from build123d import *

# Parameters (mm, degrees)
EXTRUDE_1_DEPTH     = 200
FILLET_1_R          = 80
EXTRUDE_2_DEPTH     = 100
SKETCH_3_R          = 25
CUT_EXTRUDE_1_DEPTH = 160
EXTRUDE_START       = 12
SKETCH_4_R          = 25
EXTRUDE_3_DEPTH     = 12
SKETCH_5_R          = 28
EXTRUDE_4_DEPTH     = 4
SKETCH_6_R          = 20
EXTRUDE_5_DEPTH     = 10
CHAMFER_1_SIZE2     = 5
CHAMFER_1_SIZE      = 10
SKETCH_7_R          = 7
CUT_EXTRUDE_2_DEPTH = 200


with BuildPart() as part:
    # 草图1 → 凸台-拉伸1 (new body)
    with BuildSketch(Plane.XY):
        with BuildLine():
            ThreePointArc((11.613593767, -48.632545068), (50, 0), (11.613593767, 48.632545068))
            Line((11.613593767, 48.632545068), (-48.23619118, 62.924848473))
            Line((-48.23619118, 62.924848473), (-177.193873283, 39.347785035))
            ThreePointArc((-177.193873283, 39.347785035), (-210, 0), (-177.193873283, -39.347785035))
            Line((-177.193873283, -39.347785035), (-48.23619118, -62.924848473))
            Line((-48.23619118, -62.924848473), (11.613593767, -48.632545068))
        make_face()
    extrude(amount=EXTRUDE_1_DEPTH)

    # 圆角1
    fillet_1_edges = [part.edges().sort_by_distance(p)[0] for p in [
        (-48.23619118, -62.924848473, 100),
        (-48.23619118, 62.924848473, 100),
    ]]
    fillet(fillet_1_edges, radius=FILLET_1_R)

    # 草图2 → 凸台-拉伸2 (add)
    with BuildSketch(Plane.XY.offset(200)):
        with BuildLine():
            ThreePointArc((-125, 0), (-132.32233047, 17.67766953), (-150, 25))
            Line((-150, 25), (-150, -25))
            ThreePointArc((-150, -25), (-132.32233047, -17.67766953), (-125, 0))
        make_face()
        with BuildLine():
            Line((-150, -25), (-150, 25))
            ThreePointArc((-150, 25), (-175, 0), (-150, -25))
        make_face()
        with BuildLine():
            Line((-90, 25), (-150, 25))
            ThreePointArc((-150, 25), (-132.32233047, 17.67766953), (-125, 0))
            ThreePointArc((-125, 0), (-132.32233047, -17.67766953), (-150, -25))
            Line((-150, -25), (-90, -25))
            ThreePointArc((-90, -25), (-115, 0), (-90, 25))
        make_face()
        with BuildLine():
            ThreePointArc((-65, 0), (-72.32233047, 17.67766953), (-90, 25))
            Line((-90, 25), (-90, -25))
            ThreePointArc((-90, -25), (-72.32233047, -17.67766953), (-65, 0))
        make_face()
        with BuildLine():
            Line((-90, -25), (-90, 25))
            ThreePointArc((-90, 25), (-115, 0), (-90, -25))
        make_face()
    extrude(amount=EXTRUDE_2_DEPTH)

    # 草图3 → 切除-拉伸1 (cut)
    with BuildSketch(Plane(origin=(0, 0, 0), x_dir=(-1, 0, 0), z_dir=(0, 0, -1))):
        Circle(SKETCH_3_R)
    extrude(amount=-CUT_EXTRUDE_1_DEPTH, mode=Mode.SUBTRACT)

    # 草图4 → 凸台-拉伸3 (add)
    with BuildSketch(Plane(origin=(0, 0, 0), x_dir=(-1, 0, 0), z_dir=(0, 0, -1)).offset(EXTRUDE_START)):
        with Locations(Location((150, 0, 0), (0, 0, 180))):
            Circle(SKETCH_4_R)
    extrude(amount=-EXTRUDE_3_DEPTH)

    # 草图5 → 凸台-拉伸4 (add)
    with BuildSketch(Plane(origin=(0, 0, -12), x_dir=(-1, 0, 0), z_dir=(0, 0, -1))):
        with Locations((150, 0)):
            Circle(SKETCH_5_R)
    extrude(amount=EXTRUDE_4_DEPTH)

    # 草图6 → 凸台-拉伸5 (add)
    with BuildSketch(Plane(origin=(0, 0, -16), x_dir=(-1, 0, 0), z_dir=(0, 0, -1))):
        with Locations((150, 0)):
            Circle(SKETCH_6_R)
    extrude(amount=EXTRUDE_5_DEPTH)

    # 倒角1
    chamfer_1_edges = [part.edges().sort_by_distance(p)[0] for p in [
        (-130, 0, -26),
    ]]
    chamfer_1_side = [part.faces().sort_by_distance(p)[0] for p in [
        (-130, 0, -25.9),
    ]]
    chamfer(chamfer_1_edges, length=CHAMFER_1_SIZE - 0.0001, length2=CHAMFER_1_SIZE2 - 0.0001, reference=chamfer_1_side[0])  # a hair under: the kernel refuses the full size

    # 草图7 → 切除-拉伸2 (cut)
    with BuildSketch(Plane(origin=(0, 0, -26), x_dir=(-1, 0, 0), z_dir=(0, 0, -1))):
        with Locations((150, 0)):
            Circle(SKETCH_7_R)
    extrude(amount=-CUT_EXTRUDE_2_DEPTH, mode=Mode.SUBTRACT)


solid = part.part
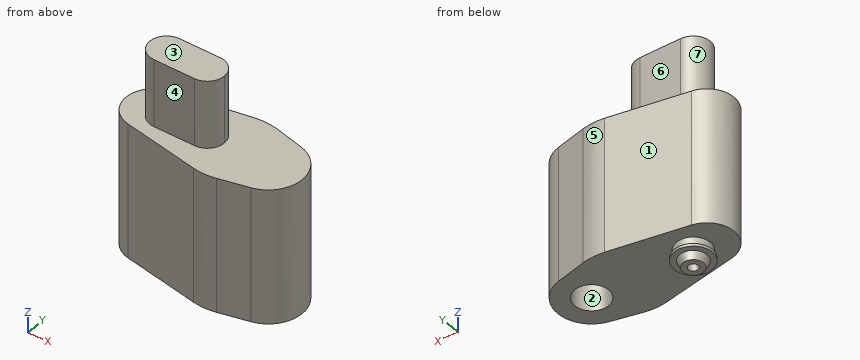
Design review of the part built by this model. Coordinates are the model's own, in mm. Face numbers are marked on the shaded views. A direction names the side the tool comes from. Coordinates: 2 decimals unless noted, no trailing zeros. Loops run counter-clockwise (first coordinate to the right, second up) from the corner with the lowest first, then second, coordinate; pieces in that order, holes last. Notation, with made-up numbers: (6.25, -2) - (27.25, -2) arc R12 cw to (27.25, 10) - close; hole circle Ø6 at (76, 31). An arc over 180 degrees is marked (long way). Use CSV: the item, a comma, the result in double quotes. Start each with the question number.
1. Clearance check with flat-ended pins moving along their axes: pin 1 (18 mm diameter, centred on x = -133, z = 248.5, fed in from -Y); pin 2 (15.5 mm diameter, centred on x = -147, y = 3, fed in from -Z); pin 3 (25 mm diameter, centred on x = -8, y = 0.5, fed in from -Z); pin 4 (6 mm diameter, centred on x = -62, z = 179.5, fed in from -Y). State where each tip first meets the part, or that it passes through.
2. Add section D-D on y = -33. Give the boundary of the cut face in (x, z), plus the area to 3 significant figures.
3. Add section C-C on x = -100.5. Give the boundary of the cut face in (y, z).
4. Add section B-B on x = 0. Give the boundary of the cut face in (y, z), plus the area to 3 significant figures.
5. For the marked faces 5, 6 and 7, list the 3-axis set-ups (+Z, -Z, +X, -X, +Y, -Y) from which the entire face can be reached by the end or side of a thin tool; tool diameter is ignored.
6. To check wall thickness, follow probe 1 along Z at (x, y) = (-193, 26.5); probe 2 along Y at (x, z) = (-150, 83.5); probe 3 along X at (y, z) = (4.5, 77). State the ranges of each line that lie inside material, in increasing order.
7. Mouldability with a two-part tool opening along Y and no side actions: class the marked faces 1, 2, 3 and 4 as released by +Y, released by -Y, zero draft, split by the parting line, or undercut.
8. Add section A-A on z = 17. Give the boundary of the cut face in (x, y).
Resolved:
1,pin 1,"y = -25"
1,pin 2,"z = -26"
1,pin 3,"z = 160"
1,pin 4,"y = -60.74"
2,outline,"(-192.61, 0) - (37.56, 0) - (37.56, 200) - (-192.61, 200) - close"
2,area,"46,000 mm2"
3,outline,"(-53.37, 0) - (53.37, 0) - (53.37, 200) - (25, 200) - (25, 300) - (-25, 300) - (-25, 200) - (-53.37, 200) - close"
4,outline,"(-51.41, 0) - (-25, 0) - (-25, 160) - (25, 160) - (25, 0) - (51.41, 0) - (51.41, 200) - (-51.41, 200) - close"
4,area,"12,600 mm2"
5,face 5,"+Z, -Z, +Y"
5,face 6,"+Z, +X, -X, +Y"
5,face 7,"+Z, -X"
6,probe 1,"0 to 200"
6,probe 2,"-44.32 to -7, 7 to 44.32"
6,probe 3,"-209.75 to -155.36, -144.64 to -24.59, 24.59 to 49.8"
7,face 1,"released by +Y"
7,face 2,"undercut"
7,face 3,"zero draft"
7,face 4,"released by -Y"
8,outline,"(-177.19, -39.35) - (-64.81, -59.89) arc R80 ccw to (-31.84, -59.01) - (11.61, -48.63) arc R50 ccw to (11.61, 48.63) - (-31.84, 59.01) arc R80 ccw to (-64.81, 59.89) - (-177.19, 39.35) arc R40 ccw to start; hole circle Ø14 at (-150, 0); hole circle Ø50 at (0, 0)"
